Could you check a few things on this model? Use its own coordinates, in mm. A direction names the side the tool comes from. Give positions to 0.01 mm unless a question says otherwise; leave off trailing zeros. Write each loop counter-clockwise with the first axis right and the second up, starting at its lowest first coordinate (ties: lowest second). Pieces come first, ordered by that corner, then holes. Notation, with made-up numbers: (-26, 8.5) -> (-4, 8.5) arc R16 cw to (-4, 12.5) -> close; hole circle Ø11 at (70.5, -36.75). An arc over 180 degrees is marked (long way). Write item = value, one per line. Start each with the question number.
```python
from build123d import *

# Parameters (mm, degrees)
SKETCH1_W           = 120
SKETCH1_H           = 60
BOSS_EXTRUDE1_DEPTH = 50
SKETCH2_W           = 114
SKETCH2_H           = 54
CUT_EXTRUDE1_DEPTH  = 47
SKETCH5_W           = 70
SKETCH5_H           = 24
CUT_EXTRUDE3_DEPTH  = 7
SKETCH6_W           = 4.5
SKETCH6_H           = 4.5
CUT_EXTRUDE4_DEPTH  = 7
SKETCH7_W           = 12
SKETCH7_H           = 13
SKETCH7_W_2         = 10
CUT_EXTRUDE5_DEPTH  = 3
SKETCH8_W           = 52
SKETCH8_H           = 2
CUT_EXTRUDE6_DEPTH  = 13
SKETCH9_W           = 117
SKETCH9_H           = 57
CUT_EXTRUDE7_DEPTH  = 1.5
SKETCH10_W          = 8
SKETCH10_H          = 8
CUT_EXTRUDE8_DEPTH  = 11.5


with BuildPart() as part:
    # Sketch1 → Boss-Extrude1 (new body)
    with BuildSketch(Plane(origin=(0, 0, 0), x_dir=(1, 0, 0), z_dir=(0, 1, 0))):
        Rectangle(SKETCH1_W, SKETCH1_H)
    extrude(amount=BOSS_EXTRUDE1_DEPTH)

    # Sketch2 → Cut-Extrude1 (cut)
    with BuildSketch(Plane.XZ):
        Rectangle(SKETCH2_W, SKETCH2_H)
    extrude(amount=-CUT_EXTRUDE1_DEPTH, mode=Mode.SUBTRACT)

    # Sketch5 → Cut-Extrude3 (cut)
    with BuildSketch(Plane.XY.offset(30)):
        with Locations((13, 27)):
            Rectangle(SKETCH5_W, SKETCH5_H)
    extrude(amount=-CUT_EXTRUDE3_DEPTH, mode=Mode.SUBTRACT)

    # Sketch6 → Cut-Extrude4 (cut)
    with BuildSketch(Plane.XY.offset(30)):
        with Locations((-47.75, 22.25)):
            Rectangle(SKETCH6_W, SKETCH6_H)
    extrude(amount=-CUT_EXTRUDE4_DEPTH, mode=Mode.SUBTRACT)

    # Sketch7 → Cut-Extrude5 (cut)
    with BuildSketch(Plane(origin=(60, 0, 0), x_dir=(0, 0, -1), z_dir=(1, 0, 0))):
        with Locations((-11, 6.5)):
            Rectangle(SKETCH7_W, SKETCH7_H)
        with Locations((19, 6.5)):
            Rectangle(SKETCH7_W_2, SKETCH7_H)
    extrude(amount=-CUT_EXTRUDE5_DEPTH, mode=Mode.SUBTRACT)

    # Sketch8 → Cut-Extrude6 (cut)
    with BuildSketch(Plane(origin=(60, 0, 0), x_dir=(0, 0, -1), z_dir=(1, 0, 0))):
        Rectangle(SKETCH8_W, SKETCH8_H)
    extrude(amount=-CUT_EXTRUDE6_DEPTH, mode=Mode.SUBTRACT)

    # Sketch9 → Cut-Extrude7 (cut)
    with BuildSketch(Plane.XZ):
        Rectangle(SKETCH9_W, SKETCH9_H)
    extrude(amount=-CUT_EXTRUDE7_DEPTH, mode=Mode.SUBTRACT)

    # Sketch10 → Cut-Extrude8 (cut)
    with BuildSketch(Plane(origin=(0, 0, -30), x_dir=(-1, 0, 0), z_dir=(0, 0, -1))):
        with Locations((0, 12)):
            Rectangle(SKETCH10_W, SKETCH10_H)
    extrude(amount=-CUT_EXTRUDE8_DEPTH, mode=Mode.SUBTRACT)


solid = part.part
```
(1) Imagine slicing it at B-B (y = 23). Please give me the cut outline in (x, z).
(2) Imagine slicing it at C-C (y = 31.5). Please give me the cut outline in (x, z), then the cut area to 3 significant figures.
(3) I'm going to push flat-ended pins straight in: pin 1 (8 mm diameter, centred on x = 44, z = 17.5, fed in from -Y); pin 2 (1 mm diameter, centred on y = 6.5, z = -15.5, fed in from +X); pin 3 (6 mm diameter, centred on x = -17.5, y = 34.5, fed in from +Z). Where does each tip first touch, or does it pass through?
(4) We'd pull the mould along X, two halves only. Please class faces 1 (the flat face through (-60, 25, 0)), 2 (the flat face through (-1, 25, -30)), 3 (the flat face through (-48, 20, 29)): released by +X, released by -X, zero draft, split by the parting line, or undercut.
(5) Imagine slicing it at D-D (z = -10). Please give me the cut outline in (x, y), then the cut area to 3 significant figures.
(6) Imagine slicing it at A-A (x = -15). Please give me the cut outline in (y, z), then the cut area to 4 significant figures.
(7) On a 3-axis mill with a long thin cutter (end or side, diameter ignored), from which of +Z, -Z, +X, -X, +Y, -Y can I reach the whole of each face in a straight line? I mean faces 4 (the flat face through (-1, 24, -27)), 5 (the flat face through (59, 7, -24)), 6 (the flat face through (-4, 12, -29)). Say none if no direction works.
(8) If I drill on line 1 along X through (y, z) = (2, 26); line 2 along Z through (x, y) = (-2.5, 4); line 3 along Y through (x, z) = (-34.5, -15), over which ranges is the centre line in solid material (lowest first)? Write a range as from..to.
Answers below:
q1.outline = (-60, -30) -> (60, -30) -> (60, 30) -> (48, 30) -> (48, 27) -> (57, 27) -> (57, -27) -> (-57, -27) -> (-57, 27) -> (-50, 27) -> (-50, 30) -> (-60, 30) -> close; (-45.5, 27) -> (-22, 27) -> (-22, 30) -> (-45.5, 30) -> close
q2.outline = (-60, -30) -> (60, -30) -> (60, 30) -> (48, 30) -> (48, 27) -> (57, 27) -> (57, -27) -> (-57, -27) -> (-57, 27) -> (-22, 27) -> (-22, 30) -> (-60, 30) -> close
q2.area = 834 mm^2
q3.pin_1 = 47
q3.pin_2 = -57
q3.pin_3 = -27
q4.face_1 = released by -X
q4.face_2 = zero draft
q4.face_3 = undercut
q5.outline = (-60, 0) -> (-58.5, 0) -> (-58.5, 1.5) -> (-57, 1.5) -> (-57, 47) -> (57, 47) -> (57, 1.5) -> (58.5, 1.5) -> (58.5, 1) -> (60, 1) -> (60, 50) -> (-60, 50) -> close
q5.area = 636 mm^2
q6.outline = (0, -30) -> (50, -30) -> (50, 30) -> (39, 30) -> (39, 27) -> (47, 27) -> (47, -27) -> (1.5, -27) -> (1.5, -28.5) -> (0, -28.5) -> close; (0, 28.5) -> (1.5, 28.5) -> (1.5, 27) -> (15, 27) -> (15, 30) -> (0, 30) -> close
q6.area = 385.5 mm^2
q7.face_4 = -Y
q7.face_5 = +X, -Y
q7.face_6 = -Z
q8.line_1 = -60..-57, 57..60
q8.line_2 = -30..-27, 27..30
q8.line_3 = 47..50
